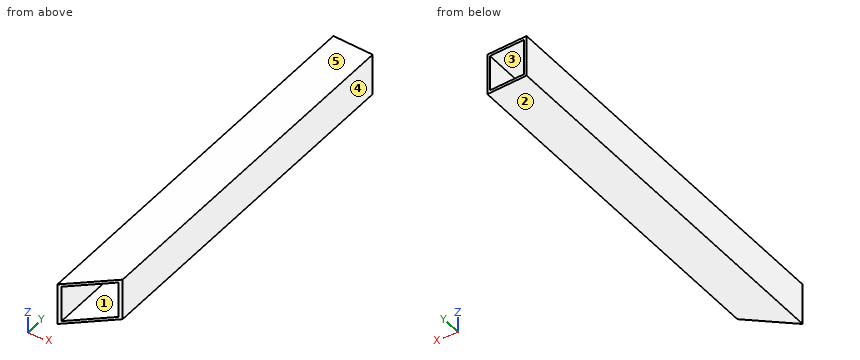
```python
from build123d import *

# Parameters (mm, degrees)
SKETCH4_W           = 25.4
SKETCH4_H           = 25.4
BOSS_EXTRUDE1_DEPTH = 252.579
CUT_EXTRUDE1_DEPTH  = 256.120503372
CUT_EXTRUDE2_DEPTH  = 256.120503372
SHELL1_T            = -1.651


with BuildPart() as part:
    # Sketch4 → Boss-Extrude1 (new body)
    with BuildSketch(Plane(origin=(0, 0, 0), x_dir=(1, 0, 0), z_dir=(0, 1, 0))):
        with Locations((12.7, 12.7)):
            Rectangle(SKETCH4_W, SKETCH4_H)
    extrude(amount=BOSS_EXTRUDE1_DEPTH)

    # Sketch5 → Cut-Extrude1 (cut, through all)
    with BuildSketch(Plane.XY):
        Polygon((0, 252.579), (25.4, 252.579), (25.4, 250.759583461), align=None)
    extrude(amount=-CUT_EXTRUDE1_DEPTH, mode=Mode.SUBTRACT)

    # Sketch6 → Cut-Extrude2 (cut, through all)
    with BuildSketch(Plane.XY):
        Polygon((0, 0), (25.4, 22.004395982), (25.4, 0), align=None)
    extrude(amount=-CUT_EXTRUDE2_DEPTH, mode=Mode.SUBTRACT)

    # Shell1
    shell1_openings = [part.faces().sort_by_distance(p)[0] for p in [
        (12.7, 251.669291731, -12.7),
        (12.7, 11.002197991, -12.7),
    ]]
    offset(amount=SHELL1_T, openings=shell1_openings, kind=Kind.INTERSECTION)


solid = part.part
```
Could you check a few things on this model? Use its own coordinates, in mm. Face numbers are marked on the shaded views. A direction names the side the tool comes from. Round coordinates to 2 decimals unless told otherwise and drop trailing zeros. Loops run counter-clockwise (first coordinate to the right, second up) from the corner with the lowest first, then second, coordinate; pieces in that order, holes last. Notation, with made-up numbers: (-1, 16) - (17, 16) arc R20 ccw to (17, 31) - close; hole circle Ø6 at (17, -5). An arc over 180 degrees is marked (long way). Answer as CSV lines item,"result".
1. Please list where these lines run through material, in increasing order: line 1 along Z through (x, y) = (6.5, 180); line 2 along X through (y, z) = (106, -7.75); line 3 along X through (y, z) = (12, -1.75). Write a range as [from, to].
Filled in:
line 1,"z = [-25.4, -23.75], [-1.65, 0]"
line 2,"x = [0, 1.65], [23.75, 25.4]"
line 3,"x = [0, 1.65]"
2. I want a section at C-C on y = 115. List the corners of the cut face in (x, z) for me, then the cut area to 3 significant figures.
Filled in:
outline,"(0, -25.4) - (25.4, -25.4) - (25.4, 0) - (0, 0) - close; hole (1.65, -23.75) - (23.75, -23.75) - (23.75, -1.65) - (1.65, -1.65) - close"
area,"157 mm^2"
3. I want a section at A-A on z = -8.5. List the corners of the cut face in (x, y) for me.
Filled in:
outline,"(0, 0) - (1.65, 1.43) - (1.65, 252.46) - (0, 252.58) - close; (23.75, 20.57) - (25.4, 22) - (25.4, 250.76) - (23.75, 250.88) - close"
4. I want a section at B-B on x = 10. List the corners of the cut face in (y, z) for me.
Filled in:
outline,"(8.66, -25.4) - (251.86, -25.4) - (251.86, -23.75) - (8.66, -23.75) - close; (8.66, -1.65) - (251.86, -1.65) - (251.86, 0) - (8.66, 0) - close"
5. On a 3-axis mill with a long thin cutter (end or side, diameter ignored), from which of +Z, -Z, +X, -X, +Y, -Y can I reach the whole of each face in a straight line? I mean the marked faces 1 and 2. Say none if no direction works.
Filled in:
face 1,"+Y, -Y"
face 2,"-Z, +X, -X, +Y, -Y"
6. We'd pull the mould along X, two halves only. Please class the marked faces 3, 4 and 5: +X half, -X half, draft (parallel to the pull), parting line (faces both ways), or undercut.
Filled in:
face 3,"undercut"
face 4,"+X half"
face 5,"draft"
